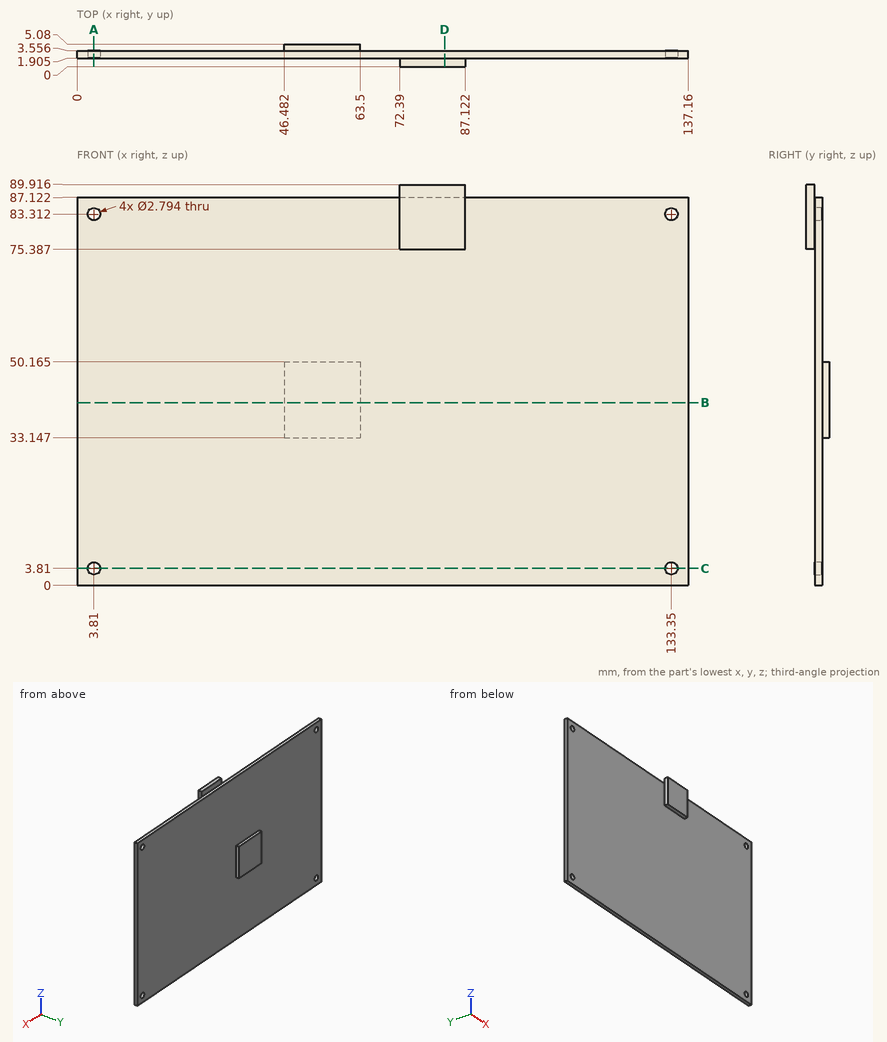
Input: dimensioned drawing with shaded views. Units: mm. Origin: part minimum x, y, z. Give positions to 0.01 mm unless a question says otherwise; leave off trailing zeros. Write each loop counter-clockwise with the first axis right and the second up, starting at its lowest first coordinate (ties: lowest second). Pieces come first, ordered by that corner, then holes. Notation, with made-up numbers: M -24,29 L -12,29 A35 ccw -12,67 Z; hole C 87,67.5 d1. An arc over 180 degrees is marked long. Return JSON: item names as keys, results as strings. Group by question number.
1) Material intervals for line 1 along X through (y, z) = (3.25, 3.81); line 2 along Z through (x, y) = (133.35, 2.3) (3 decimals); line 3 along Y through (x, z) = (114.5, 64.5) (3 decimals), sorted ascending. Write a range as [from, to].
2) Cut plane B-B, the plane z = 41. Output: boundary loops of the cut face in (x, y) (3 decimals), plus the area to 3 significant figures.
3) Pin query (flat end, axial travel): P1, Ø1.7, axis at x = 133.35, z = 83.312, coming from the +Y side; P2, Ø1, axis at x = 81.5, y = 0.5, coming from the -Z side; P3, Ø6, axis at x = 97, z = 15.5, coming from the +Y side; P4, Ø2, axis at y = 0.5, z = 85, coming from the -X side. Return the tip coordinate at first contact, or that it passes through.
4) Cut plane C-C, the plane z = 3.81. Output: boundary loops of the cut face in (x, y) (3 decimals), plus the area to 3 significant figures.
5) Cut plane D-D, the plane x = 82.5. Output: boundary loops of the cut face in (y, z) (1 decimal).
6) Cut plane A-A, the plane x = 3.81. Output: boundary loops of the cut face in (y, z) (3 decimals), plus the area to 3 significant figures.
Recorded:
{
 "1": {"line 1": "x = [0, 2.41], [5.21, 131.95], [134.75, 137.16]", "line 2": "z = [0, 2.413], [5.207, 81.915], [84.709, 87.122]", "line 3": "y = [1.905, 3.556]"},
 "2": {"outline": "M 0,1.905 L 137.16,1.905 L 137.16,3.556 L 63.5,3.556 L 63.5,5.08 L 46.482,5.08 L 46.482,3.556 L 0,3.556 Z", "area": "252 mm²"},
 "3": {"P1": "passes through", "P2": "stops at z = 75.39", "P3": "stops at y = 3.56", "P4": "stops at x = 72.39"},
 "4": {"outline": "M 0,1.905 L 2.413,1.905 L 2.413,3.556 L 0,3.556 Z; M 5.207,1.905 L 131.953,1.905 L 131.953,3.556 L 5.207,3.556 Z; M 134.747,1.905 L 137.16,1.905 L 137.16,3.556 L 134.747,3.556 Z", "area": "217 mm²"},
 "5": {"outline": "M 0,75.4 L 1.9,75.4 L 1.9,0 L 3.6,0 L 3.6,87.1 L 1.9,87.1 L 1.9,89.9 L 0,89.9 Z"},
 "6": {"outline": "M 1.905,0 L 3.556,0 L 3.556,2.413 L 1.905,2.413 Z; M 1.905,5.207 L 3.556,5.207 L 3.556,81.915 L 1.905,81.915 Z; M 1.905,84.709 L 3.556,84.709 L 3.556,87.122 L 1.905,87.122 Z", "area": "135 mm²"}
}
